CAD build for the part. Positions are in the model's coordinates, mm. Face numbers are marked on the shaded views. A direction names the side the tool comes from. Round coordinates to 2 decimals unless told otherwise and drop trailing zeros. Order: outer loops, then holes, each group sorted by start corner. A loop starts at its lowest first (then second) coordinate and runs counter-clockwise, first axis right, second up. Notation, with made-up numbers: M -23,17 L 31,17 A28 ccw 31,48 Z; hole C -35,-22.75 d6. An arc over 180 degrees is marked long. Answer as CSV lines item,"result". Start each with the question number.
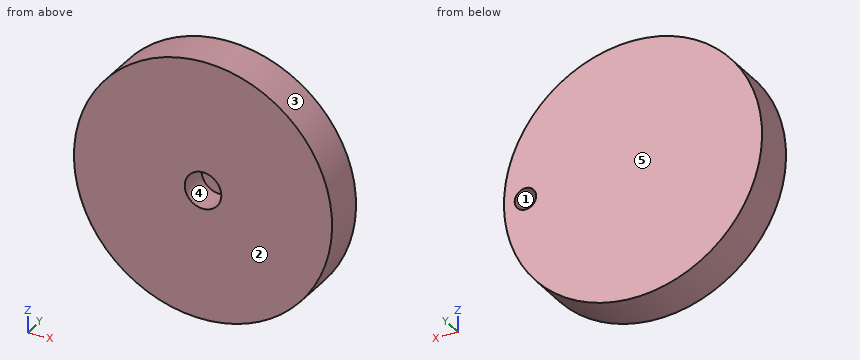
```python
from build123d import *

# Parameters (mm, degrees)
SKETCH1_R           = 30
BOSS_EXTRUDE1_DEPTH = 10
SKETCH2_R           = 4.25
CUT_EXTRUDE1_DEPTH  = 7
SKETCH3_R           = 2.5
CUT_EXTRUDE2_DEPTH  = 6


with BuildPart() as part:
    # Sketch1 → Boss-Extrude1 (new body)
    with BuildSketch(Plane(origin=(0, 0, 0), x_dir=(1, 0, 0), z_dir=(0, 1, 0))):
        with Locations(Location((0, 0, 0), (0, 0, 270))):
            Circle(SKETCH1_R)
    extrude(amount=BOSS_EXTRUDE1_DEPTH)

    # Sketch2 → Cut-Extrude1 (cut)
    with BuildSketch(Plane.XZ):
        with Locations(Location((0, 0, 0), (0, 0, 270))):
            Circle(SKETCH2_R)
    extrude(amount=-CUT_EXTRUDE1_DEPTH, mode=Mode.SUBTRACT)

    # Sketch3 → Cut-Extrude2 (cut)
    with BuildSketch(Plane(origin=(0, 10, 0), x_dir=(1, 0, 0), z_dir=(0, 1, 0))):
        with Locations(Location((25, 0, 0), (0, 0, 270))):
            Circle(SKETCH3_R)
    extrude(amount=-CUT_EXTRUDE2_DEPTH, mode=Mode.SUBTRACT)


solid = part.part
```
Q1. Tool access for the marked faces 1 and 2: list every direction of +Z, -Z, +X, -X, +Y, -Y with a clear straight run to the whole face (end or side of a thin tool).
Q2. Band-saw the part on A-A, the plane z = 0. Write the cut outline in (x, y), then the cut area to 4 significant figures.
Q3. Band-saw the part on D-D, the plane y = 8.25. Write the cut outline in (x, z).
Q4. Mould opens along X. For the marked faces 3, 4 and 5 say: +X half, -X half, draft (parallel to the pull), parting line (faces both ways), or undercut.
Q5. Drop flat-ended pins along their axis: P1, Ø4, axis at x = 19, y = 6, coming from the +Z side; P2, Ø1.5, axis at x = 25.5, z = 0.5, coming from the +Y side; P3, Ø6, axis at x = -16.5, z = -9, coming from the -Y side; P4, Ø3, axis at x = -17, y = 1, coming from the -Z side. Give the stop position or say it passes through.
Q6. Probe line 1 along X through (y, z) = (5.95, 0); line 2 along X through (y, z) = (7.3, 0); line 3 along X through (y, z) = (1.75, 0). List the from-to ranges inside material, lowest first. Write a range as from..to.
Q7. Band-saw the part on B-B, the plane x = 0. Write the cut outline in (y, z), then the cut area to 4 significant figures.
Q8. Band-saw the part on C-C, the plane y = 2.75. Write the cut outline in (x, z), then the cut area to 3 significant figures.
Answer:
1,face 1,"+Y"
1,face 2,"+Z, -Z, +X, -X, -Y"
2,outline,"M -30,0 L -4.25,0 L -4.25,7 L 4.25,7 L 4.25,0 L 30,0 L 30,10 L 27.5,10 L 27.5,4 L 22.5,4 L 22.5,10 L -30,10 Z"
2,area,"510.5 mm^2"
3,outline,"C 0,0 d60; hole C 25,0 d5"
4,face 3,"parting line"
4,face 4,"undercut"
4,face 5,"draft"
5,P1,"stops at z = 24.72"
5,P2,"stops at y = 4"
5,P3,"stops at y = 0"
5,P4,"stops at z = -25.69"
6,line 1,"x = -30..-4.25, 4.25..22.5, 27.5..30"
6,line 2,"x = -30..22.5, 27.5..30"
6,line 3,"x = -30..-4.25, 4.25..30"
7,outline,"M 0,-30 L 10,-30 L 10,30 L 0,30 L 0,4.25 L 7,4.25 L 7,-4.25 L 0,-4.25 Z"
7,area,"540.5 mm^2"
8,outline,"C 0,0 d60; hole C 0,0 d8.5"
8,area,"2,770 mm^2"
